Source: CAD feature listing. Evaluate the final solid. Frame: model axes, mm. Give positions to 0.01 mm unless a question says otherwise; leave off trailing zeros. Order: outer loops, then holes, each group sorted by start corner. A loop starts at its lowest first (then second) coordinate and runs counter-clockwise, first axis right, second up.
1) Section A-A, the plane y = 46.99. Return loops of the section in (x, z), plus the area to 3 significant figures.
2) First-contact query: P1, Ø12, axis at x = -2, y = 42.5, coming from the -Z side; P2, Ø1.8, axis at x = 24.13, y = -24.13, coming from the +Z side. Flat tips, straight axial feed; report the tip coordinate or a pass-through.
3) Material intervals for line 1 (X direction, y = 46.99, z = 0.8); line 2 (Y direction, x = 24.13, z = 1.3); line 3 (Y direction, x = 24.13, z = 3.25), sorted ascending.
4) Section B-B, the plane x = 24.13. Return loops of the section in (y, z).
```python
from build123d import *

# Parameters (mm, degrees)
SKETCH1_W           = 81.28
SKETCH1_H           = 81.28
SKETCH1_R           = 1.524
BOSS_EXTRUDE1_DEPTH = 5.08
SKETCH2_R           = 2.667
CUT_EXTRUDE1_DEPTH  = 2.54
SKETCH3_W           = 81.28
SKETCH3_H           = 81.28
SKETCH3_W_2         = 80.264
SKETCH3_H_2         = 80.264
CUT_EXTRUDE2_DEPTH  = 74.813116721


with BuildPart() as part:
    # Sketch1 → Boss-Extrude1 (new body)
    with BuildSketch(Plane.XY):
        with Locations((-11.43, 11.43)):
            Rectangle(SKETCH1_W, SKETCH1_H)
        with Locations(Location((-46.99, 46.99, 0), (0, 0, 180))):
            Circle(SKETCH1_R, mode=Mode.SUBTRACT)
        with Locations(Location((-46.99, -24.13, 0), (0, 0, 180))):
            Circle(SKETCH1_R, mode=Mode.SUBTRACT)
        with Locations(Location((24.13, -24.13, 0), (0, 0, 180))):
            Circle(SKETCH1_R, mode=Mode.SUBTRACT)
        with Locations(Location((24.13, 46.99, 0), (0, 0, 180))):
            Circle(SKETCH1_R, mode=Mode.SUBTRACT)
    extrude(amount=BOSS_EXTRUDE1_DEPTH)

    # Sketch2 → Cut-Extrude1 (cut)
    with BuildSketch(Plane.XY.offset(5.08)):
        with Locations((-46.99, -24.13)):
            Circle(SKETCH2_R)
        with Locations((-46.99, 46.99)):
            Circle(SKETCH2_R)
        with Locations((24.13, 46.99)):
            Circle(SKETCH2_R)
        with Locations((24.13, -24.13)):
            Circle(SKETCH2_R)
    extrude(amount=-CUT_EXTRUDE1_DEPTH, mode=Mode.SUBTRACT)

    # Sketch3 → Cut-Extrude2 (cut, through all)
    with BuildSketch(Plane.XY.offset(5.08)):
        with Locations((-11.43, 11.43)):
            Rectangle(SKETCH3_W, SKETCH3_H)
        with Locations((-11.43, 11.43)):
            Rectangle(SKETCH3_W_2, SKETCH3_H_2, mode=Mode.SUBTRACT)
    extrude(amount=-CUT_EXTRUDE2_DEPTH, mode=Mode.SUBTRACT)


solid = part.part
```
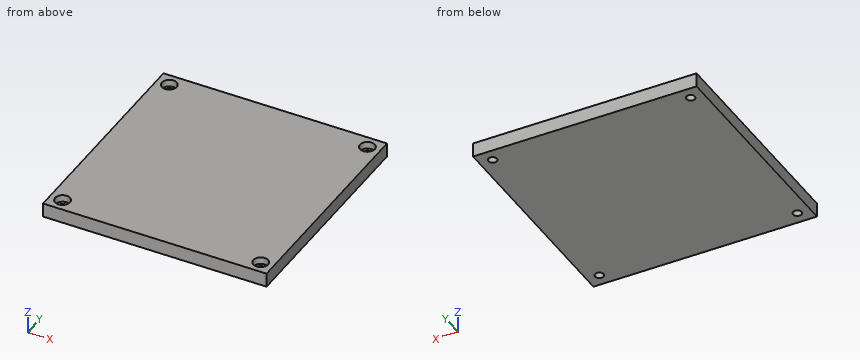
From the geometry:
1. outline: (-51.56, 0) - (-48.51, 0) - (-48.51, 2.54) - (-49.66, 2.54) - (-49.66, 5.08) - (-51.56, 5.08) - close; (-45.47, 0) - (22.61, 0) - (22.61, 2.54) - (21.46, 2.54) - (21.46, 5.08) - (-44.32, 5.08) - (-44.32, 2.54) - (-45.47, 2.54) - close; (25.65, 0) - (28.7, 0) - (28.7, 5.08) - (26.8, 5.08) - (26.8, 2.54) - (25.65, 2.54) - close
1. area: 365 mm2
2. P1: stops at z = 0
2. P2: passes through
3. line 1: x = -51.56 to -48.51, -45.47 to 22.61, 25.65 to 28.7
3. line 2: y = -28.7 to -25.65, -22.61 to 45.47, 48.51 to 51.56
3. line 3: y = -28.7 to -26.8, -21.46 to 44.32, 49.66 to 51.56
4. outline: (-28.7, 0) - (-25.65, 0) - (-25.65, 2.54) - (-26.8, 2.54) - (-26.8, 5.08) - (-28.7, 5.08) - close; (-22.61, 0) - (45.47, 0) - (45.47, 2.54) - (44.32, 2.54) - (44.32, 5.08) - (-21.46, 5.08) - (-21.46, 2.54) - (-22.61, 2.54) - close; (48.51, 0) - (51.56, 0) - (51.56, 5.08) - (49.66, 5.08) - (49.66, 2.54) - (48.51, 2.54) - close
